Read the model definition and answer for the solid it produces. Units are mm, in the model's axes. Face numbers are marked on the shaded views. A direction names the side the tool comes from. Give positions to 0.01 mm unless a question says otherwise; leave off trailing zeros. Write each loop counter-clockwise with the first axis right and the second up, starting at its lowest first coordinate (ties: lowest second). Pieces come first, ordered by that corner, then holes. Notation, with made-up numbers: (54.5, -24.75) - (100.5, -24.75) arc R30 cw to (100.5, 2.25) - close; hole circle Ø1 at (57, 61.5). An arc over 180 degrees is marked (long way). Answer as CSV lines item,"result".
```python
from build123d import *

# Parameters (mm, degrees)
SKETCH3_R          = 1.5
CUT_EXTRUDE1_DEPTH = 218.944947177
SKETCH4_R          = 30
CUT_EXTRUDE2_DEPTH = 15
SKETCH5_W          = 58
SKETCH5_H          = 26
CUT_EXTRUDE3_DEPTH = 216


with BuildPart() as part:
    # Sketch2 → Revolve1 (revolve)
    with BuildSketch(Plane.XY, mode=Mode.PRIVATE) as revolve1_sk:
        Polygon((0, 0), (35, 0), (43.234110893, 9.489398467), (150, 46.5), (150, 50), (50, 20), (0, 20), (0, 7.226614915), align=None)
    revolve(revolve1_sk.sketch.rotate(Axis((0, 7.226614915, 0), (0, 1, 0)), 270), axis=Axis((0, 7.226614915, 0), (0, 1, 0)))

    # Sketch3 → Cut-Extrude1 (cut, through all)
    with BuildSketch(Plane.XZ):
        with Locations(Location((0, 7, 0), (0, 0, 270))):
            Circle(SKETCH3_R)
        with Locations(Location((7, 0, 0), (0, 0, 270))):
            Circle(SKETCH3_R)
        with Locations(Location((0, -7, 0), (0, 0, 270))):
            Circle(SKETCH3_R)
        with Locations(Location((-7, 0, 0), (0, 0, 270))):
            Circle(SKETCH3_R)
    extrude(amount=-CUT_EXTRUDE1_DEPTH, mode=Mode.SUBTRACT)

    # Sketch4 → Cut-Extrude2 (cut)
    with BuildSketch(Plane.XZ):
        with Locations(Location((0, 0, 0), (0, 0, 270))):
            Circle(SKETCH4_R)
    extrude(amount=-CUT_EXTRUDE2_DEPTH, mode=Mode.SUBTRACT)

    # Sketch5 → Cut-Extrude3 (cut, through all)
    with BuildSketch(Plane.XZ.offset(-15)):
        Rectangle(SKETCH5_W, SKETCH5_H)
    extrude(amount=CUT_EXTRUDE3_DEPTH, mode=Mode.SUBTRACT)


with BuildPart() as part_1:
    # Body-Move/Copy1: moved
    add(part.part.moved(Location((0, -15, 0))))


solid = part_1.part
```
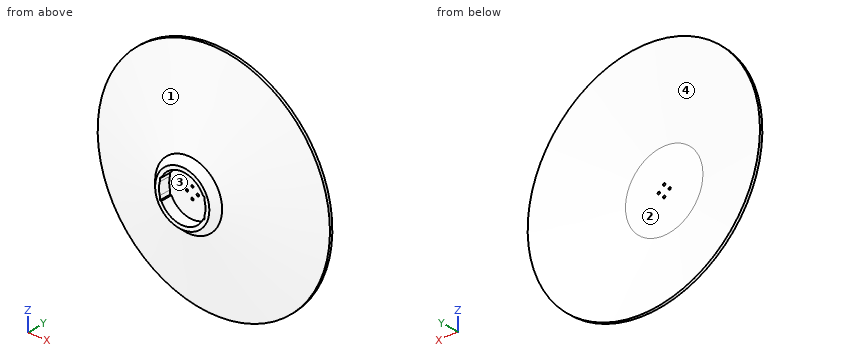
(1) For the marked faces 3 and 4, determine the directions among +Z, -Z, +X, -X, +Y, -Y from which every point of the face is accessible in a straight line to the end or side of a thin tool.
Worked out:
face 3,"-Y"
face 4,"+Y"
(2) Find the intervals of material crossed by L1, parallel to X at y = -9, z = 13.5; L2, parallel to X at y = -6, z = 10; L3, parallel to Y at x = -56, z = -7, in increasing order.
Worked out:
L1,"x = -37.87 to -26.79, 26.79 to 37.87"
L2,"x = -41.63 to -29, 29 to 41.63"
L3,"y = -0.93 to 6.93"
(3) A cutting plane is placed at A-A (y = 20.5). Write down the section's boundary in (x, z).
Worked out:
outline,"circle Ø236.54 at (0, 0); hole circle Ø203.33 at (0, 0)"
(4) Each of these flat-tipped pins is pushed along its axis until it touches: P1, Ø4, axis at x = 0, z = -7, coming from the +Y side; P2, Ø0.6, axis at x = 28.5, y = -6.5, coming from the +Z side; P3, Ø4, axis at x = -28, z = 54.5, coming from the +Y side. Where does it stop, or does it pass through?
Worked out:
P1,"stops at y = 5"
P2,"stops at z = 31.8"
P3,"stops at y = 8.98"
(5) The mould has two halves that part along X. Classify the marked faces 1 and 2: +X half, -X half, draft (parallel to the pull), parting line (faces both ways), or undercut.
Worked out:
face 1,"parting line"
face 2,"undercut"
